For this review, take the finished solid that the model builds, in its own axes (mm). Give positions to 0.01 mm unless a question says otherwise; leave off trailing zeros. Order: outer loops, then holes, each group sorted by start corner. A loop starts at its lowest first (then second) coordinate and runs counter-clockwise, first axis right, second up. Notation, with made-up numbers: M 80.5,-25 L 124.5,-25 A15 ccw 124.5,1 Z; hole C -27,-24.75 d11. An arc over 180 degrees is marked long. Use CSV: the item, a comma, the result in double quotes. Start each with the question number.
(1) Consider section A-A (y = -22). Write out the cut boundary in (x, z).
(2) Wall thickness on L1, parallel to X at y = 8.5, z = 4.85; L2, parallel to Y at x = 33, z = 2.9: over which ranges is each line inside the solid? List them lowest first. Write a range as from..to.
(3) Clearance check with flat-ended pins moving along their axes: P1, Ø1.9, axis at x = 51.02, y = -27.45, coming from the +Z side; P2, Ø5, axis at x = -51.02, y = -27.45, coming from the +Z side; P3, Ø3, axis at x = 16, z = 4, coming from the -Y side. State where each tip first meets the part, or that it passes through.
```python
from build123d import *

# Parameters (mm, degrees)
SKETCH1_W           = 108.04
SKETCH1_H           = 61.74
SKETCH1_R           = 1.6
BOSS_EXTRUDE1_DEPTH = 1.6
SKETCH2_W           = 94.57
SKETCH2_H           = 60.88
BOSS_EXTRUDE2_DEPTH = 3.55
SKETCH3_R           = 0.5
CUT_EXTRUDE1_DEPTH  = 3.55


with BuildPart() as part:
    # Sketch1 → Boss-Extrude1 (new body)
    with BuildSketch(Plane.XY):
        Rectangle(SKETCH1_W, SKETCH1_H)
        with Locations((-51.02, 27.45)):
            Circle(SKETCH1_R, mode=Mode.SUBTRACT)
        with Locations((-51.02, -27.45)):
            Circle(SKETCH1_R, mode=Mode.SUBTRACT)
        with Locations((51.02, -27.45)):
            Circle(SKETCH1_R, mode=Mode.SUBTRACT)
        with Locations((51.02, 27.45)):
            Circle(SKETCH1_R, mode=Mode.SUBTRACT)
    extrude(amount=BOSS_EXTRUDE1_DEPTH)

    # Sketch2 → Boss-Extrude2 (add)
    with BuildSketch(Plane.XY.offset(1.6)):
        with Locations((-0.015, 0)):
            Rectangle(SKETCH2_W, SKETCH2_H)
    extrude(amount=BOSS_EXTRUDE2_DEPTH)

    # Sketch3 → Cut-Extrude1 (cut)
    with BuildSketch(Plane.XY.offset(1.6)):
        with Locations((-52.02, 16.51)):
            Circle(SKETCH3_R)
        with Locations((-52.02, 13.97)):
            Circle(SKETCH3_R)
        with Locations((-52.02, 11.43)):
            Circle(SKETCH3_R)
        with Locations((-52.02, 8.89)):
            Circle(SKETCH3_R)
        with Locations((-52.02, 6.35)):
            Circle(SKETCH3_R)
        with Locations((-52.02, 3.81)):
            Circle(SKETCH3_R)
        with Locations((-52.02, 1.27)):
            Circle(SKETCH3_R)
        with Locations((-52.02, -1.27)):
            Circle(SKETCH3_R)
        with Locations((-52.02, -3.81)):
            Circle(SKETCH3_R)
        with Locations((-52.02, -6.35)):
            Circle(SKETCH3_R)
        with Locations((-52.02, -8.89)):
            Circle(SKETCH3_R)
        with Locations((-52.02, -11.43)):
            Circle(SKETCH3_R)
        with Locations((-52.02, -13.97)):
            Circle(SKETCH3_R)
        with Locations((-52.02, -16.51)):
            Circle(SKETCH3_R)
    extrude(amount=-CUT_EXTRUDE1_DEPTH, mode=Mode.SUBTRACT)


solid = part.part
```
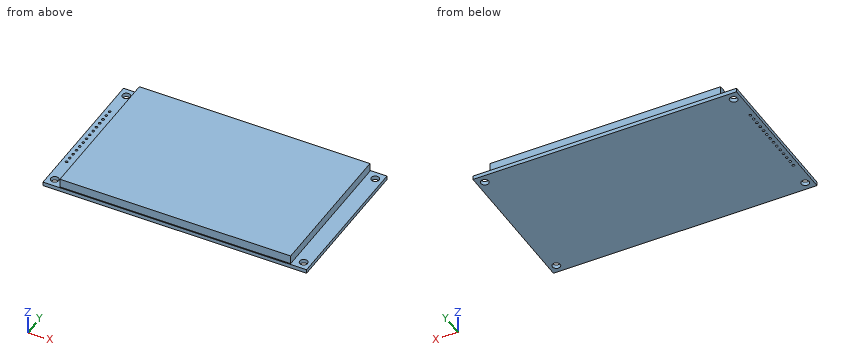
Check result:
1,outline,"M -54.02,0 L 54.02,0 L 54.02,1.6 L 47.27,1.6 L 47.27,5.15 L -47.3,5.15 L -47.3,1.6 L -54.02,1.6 Z"
2,L1,"x = -47.3..47.27"
2,L2,"y = -30.44..30.44"
3,P1,"passes through"
3,P2,"stops at z = 1.6"
3,P3,"stops at y = -30.44"
